```python
from build123d import *

# Parameters (mm, degrees)
BOSS_EXTRUDE1_DEPTH      = 4
BOSS_EXTRUDE1_DEPTH_BACK = 4


with BuildPart() as part:
    # Sketch1 → Boss-Extrude1 (new, two sides: drawn at the far end of the back side and taken through both)
    with BuildSketch(Plane(origin=(0, 0, 0), x_dir=(0, 0, -1), z_dir=(1, 0, 0)).offset(-BOSS_EXTRUDE1_DEPTH_BACK)):
        with BuildLine():
            Line((14, -15.652475842), (14, 15.652475842))
            ThreePointArc((14, 15.652475842), (0, 21), (-14, 15.652475842))
            Line((-14, 15.652475842), (-14, -15.652475842))
            ThreePointArc((-14, -15.652475842), (0, -21), (14, -15.652475842))
        make_face()
    extrude(amount=BOSS_EXTRUDE1_DEPTH + BOSS_EXTRUDE1_DEPTH_BACK)

    # Sketch2 → Cut-Revolve1 (revolve, cut)
    with BuildSketch(Plane.XY, mode=Mode.PRIVATE) as cut_revolve1_sk:
        Polygon((-4, 0), (-4, 12), (2, 12), (2, 10.5), (4, 10.5), (4, 0), align=None)
    revolve(cut_revolve1_sk.sketch.rotate(Axis((4, 0, 0), (-1, 0, 0)), 270), axis=Axis((4, 0, 0), (-1, 0, 0)), mode=Mode.SUBTRACT)

    # Sketch3 → Cut-Revolve2 (revolve, cut)
    with BuildSketch(Plane.XY, mode=Mode.PRIVATE) as cut_revolve2_sk:
        Polygon((-4, -16.5), (-4, -14), (-3.567, -14.433), (3.567, -14.433), (4, -14), (4, -16.5), align=None)
    revolve(cut_revolve2_sk.sketch.rotate(Axis((4, -16.5, 0), (-1, 0, 0)), 270), axis=Axis((4, -16.5, 0), (-1, 0, 0)), mode=Mode.SUBTRACT)

    # Sketch4 → Cut-Revolve3 (revolve, cut)
    with BuildSketch(Plane.XY, mode=Mode.PRIVATE) as cut_revolve3_sk:
        Polygon((-4, 16.5), (-4, 19), (-3.567, 18.567), (3.567, 18.567), (4, 19), (4, 16.5), align=None)
    revolve(cut_revolve3_sk.sketch.rotate(Axis((4, 16.5, 0), (-1, 0, 0)), 270), axis=Axis((4, 16.5, 0), (-1, 0, 0)), mode=Mode.SUBTRACT)


solid = part.part
```
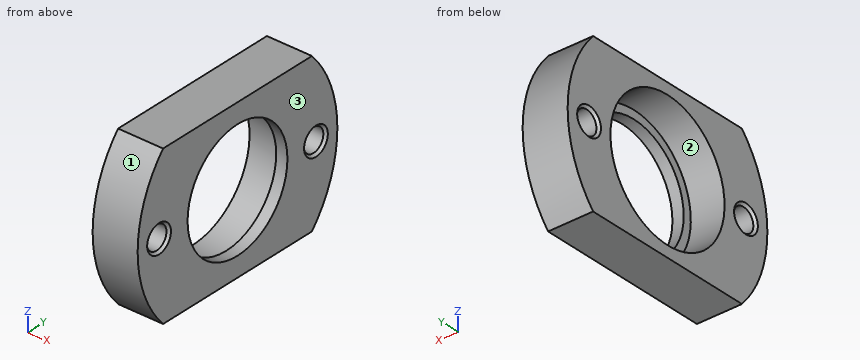
Work out the finished part from the listing and answer in its coordinate system (mm). Face numbers are marked on the shaded views. Give positions to 0.01 mm unless a question says otherwise; leave off trailing zeros. Order: outer loops, then holes, each group sorted by start corner. A loop starts at its lowest first (then second) coordinate and runs counter-clockwise, first axis right, second up.
1. Straight lines are drawn through the part: L1, parallel to Y at x = 0.75, z = 0; L2, parallel to Y at x = 2.95, z = 0; L3, parallel to Y at x = -2, z = -7. For each, find the intervals that lie inside material, in ascending order.
Result sheet:
L1: y = -21 to -18.57, -14.43 to -12, 12 to 14.43, 18.57 to 21
L2: y = -21 to -18.57, -14.43 to -10.5, 10.5 to 14.43, 18.57 to 21
L3: y = -19.8 to -9.75, 9.75 to 19.8
2. Section B-B, the plane x = -1.25 is taken. Determine the outline of the cut face in (y, z).
Result sheet:
outline: (-15.65, -14) - (15.65, -14) arc R21 ccw to (15.65, 14) - (-15.65, 14) arc R21 ccw to start; hole circle Ø4.13 at (-16.5, 0); hole circle Ø24 at (0, 0); hole circle Ø4.13 at (16.5, 0)
3. Each of these flat-tipped pins is pushed along its axis until it touches: P1, Ø2.5, axis at y = 16.5, z = 0, coming from the +X side; P2, Ø1.5, axis at x = 3, z = 9, coming from the -Y side; P3, Ø1, axis at x = 2.5, z = -8, coming from the +Y side; P4, Ø5.5, axis at y = -16.5, z = 0, coming from the -X side. Where does it stop, or does it pass through?
Result sheet:
P1: passes through
P2: stops at y = -19.31
P3: stops at y = 19.62
P4: stops at x = -4
4. Section A-A, the plane y = 0 is taken. Determine the outline of the cut face in (x, z), and give its area (3 significant figures).
Result sheet:
outline: (-4, -14) - (4, -14) - (4, -10.5) - (2, -10.5) - (2, -12) - (-4, -12) - close; (-4, 12) - (2, 12) - (2, 10.5) - (4, 10.5) - (4, 14) - (-4, 14) - close
area: 38.0 mm2
5. Section C-C, the plane z = 0 is taken. Determine the outline of the cut face in (x, y), and give its area (3 significant figures).
Result sheet:
outline: (-4, -21) - (4, -21) - (4, -19) - (3.57, -18.57) - (-3.57, -18.57) - (-4, -19) - close; (-4, -14) - (-3.57, -14.43) - (3.57, -14.43) - (4, -14) - (4, -10.5) - (2, -10.5) - (2, -12) - (-4, -12) - close; (-4, 12) - (2, 12) - (2, 10.5) - (4, 10.5) - (4, 14) - (3.57, 14.43) - (-3.57, 14.43) - (-4, 14) - close; (-4, 19) - (-3.57, 18.57) - (3.57, 18.57) - (4, 19) - (4, 21) - (-4, 21) - close
area: 83.1 mm2
6. Section D-D, the plane z = 5.5 is taken. Determine the outline of the cut face in (x, y).
Result sheet:
outline: (-4, -20.27) - (4, -20.27) - (4, -8.94) - (2, -8.94) - (2, -10.67) - (-4, -10.67) - close; (-4, 10.67) - (2, 10.67) - (2, 8.94) - (4, 8.94) - (4, 20.27) - (-4, 20.27) - close
7. The mould has two halves that part along Z. Classify the marked faces 1, 2 and 3: released by +Z, released by -Z, zero draft, split by the parting line, or undercut.
Result sheet:
face 1: split by the parting line
face 2: undercut
face 3: zero draft
